Verification items for this drawing (mm, ordinates from the low corner). A direction names the side the tool comes from. Round coordinates to 2 decimals unless told otherwise and drop trailing zeros. Loops run counter-clockwise (first coordinate to the right, second up) from the corner with the lowest first, then second, coordinate; pieces in that order, holes last. Notation, with made-up numbers: (-12, 12) - (42, 12) arc R27 ccw to (42, 45) - close; hole circle Ø5 at (-9, -10). An arc over 180 degrees is marked (long way). Write item = value, one per line.
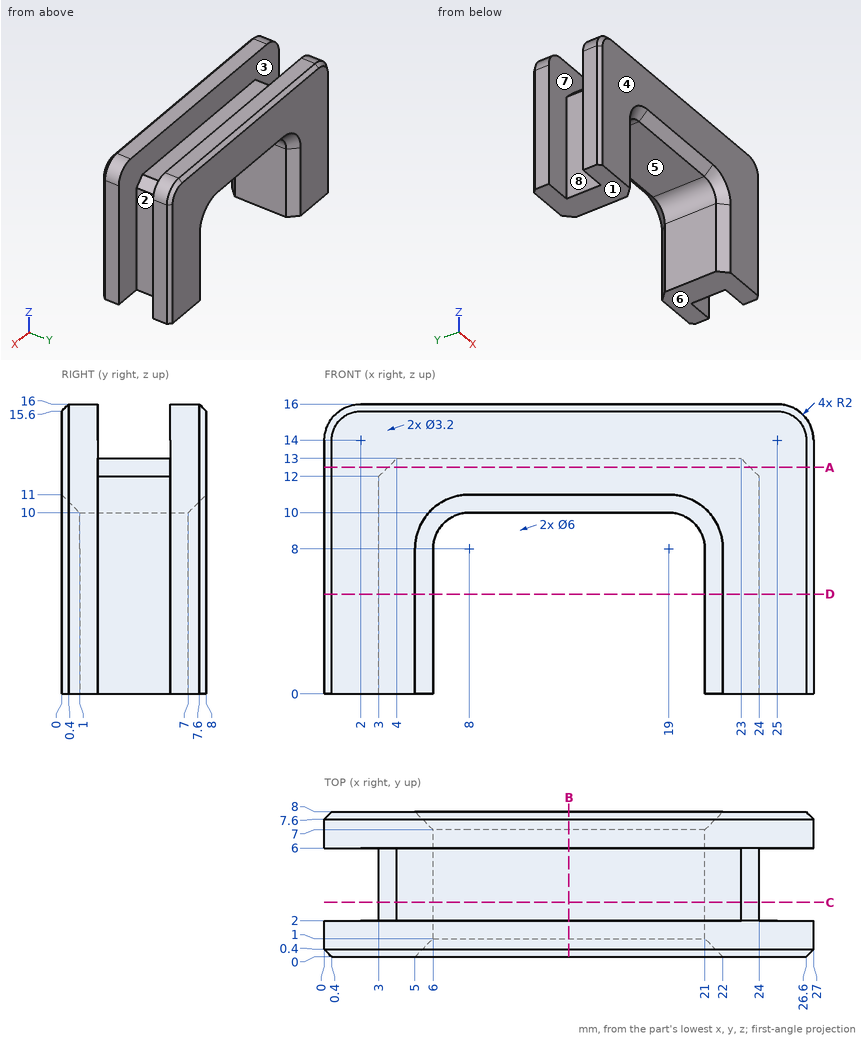
(1) Mould release check, pull along Y, two halves, no side actions. Record for the marked faces 1, 2, 3 and 4: pulls with the +Y half, pulls with the -Y half, needs draft (parallel to the pull), parting line crosses it, or undercut.
Answers follow:
face_1 = needs draft
face_2 = undercut
face_3 = undercut
face_4 = pulls with the -Y half
(2) Set-up check for the marked faces 5, 6, 7 and 8: record each of +Z, -Z, +X, -X, +Y, -Y from which the full face is reachable in a straight line by a thin tool's end or side.
Answers follow:
face_5 = -Z, +Y, -Y
face_6 = -Z, +X, -X, +Y, -Y
face_7 = +Z
face_8 = +Z, -Z, -X
(3) Section check C-C (y = 3). Enter the section's corners in (x, z), then the cut area to 3 significant figures.
Answers follow:
outline = (3, 0) - (6, 0) - (6, 8) arc R2 cw to (8, 10) - (19, 10) arc R2 cw to (21, 8) - (21, 0) - (24, 0) - (24, 12) - (23, 13) - (4, 13) - (3, 12) - close
area = 124 mm²
(4) Section check B-B (x = 13.5). Enter the section's corners in (y, z), then the cut area to 3 significant figures.
Answers follow:
outline = (0, 11) - (1, 10) - (7, 10) - (8, 11) - (8, 15.6) - (7.6, 16) - (6, 16) - (6, 13) - (2, 13) - (2, 16) - (0.4, 16) - (0, 15.6) - close
area = 34.8 mm²
(5) Gauge pin test, flat end, axial feed: pin 1 (3 mm diameter, centred on y = 4, z = 3.5, fed in from +X). Record the tip position at first contact, or that the pin passes through.
Answers follow:
pin_1 = 24
(6) Scan lines: L1, parallel to X at y = 4, z = 7.5; L2, parallel to Y at x = 2, z = 5.75; L3, parallel to X at y = 6.25, z = 2.5. Record each from-to range of solid material in increasing order. Write a range as [from, to].
Answers follow:
L1 = [3, 6], [21, 24]
L2 = [0, 2], [6, 8]
L3 = [0, 6], [21, 27]
(7) Section check D-D (z = 5.5). Enter the section's corners in (x, y), then the cut area to 3 significant figures.
Answers follow:
outline = (0, 0.4) - (0.4, 0) - (5, 0) - (6, 1) - (6, 7) - (5, 8) - (0.4, 8) - (0, 7.6) - (0, 6) - (3, 6) - (3, 2) - (0, 2) - close; (21, 1) - (22, 0) - (26.6, 0) - (27, 0.4) - (27, 2) - (24, 2) - (24, 6) - (27, 6) - (27, 7.6) - (26.6, 8) - (22, 8) - (21, 7) - close
area = 69.7 mm²
(8) Section check A-A (z = 12.5). Enter the section's corners in (x, y), then the cut area to 3 significant figures.
Answers follow:
outline = (0, 0.4) - (0.4, 0) - (26.6, 0) - (27, 0.4) - (27, 2) - (23.5, 2) - (23.5, 6) - (27, 6) - (27, 7.6) - (26.6, 8) - (0.4, 8) - (0, 7.6) - (0, 6) - (3.5, 6) - (3.5, 2) - (0, 2) - close
area = 188 mm²
